Source: CAD feature listing. Evaluate the final solid. Frame: model axes, mm. A direction names the side the tool comes from. Round coordinates to 2 decimals unless told otherwise and drop trailing zeros. Write each loop counter-clockwise with the first axis right and the second up, starting at its lowest first coordinate (ties: lowest second). Pieces come first, ordered by that corner, then holes. Notation, with made-up numbers: (23, 42.5) -> (43, 42.5) arc R22 ccw to (43, 70.5) -> close; hole circle Ø7 at (46.5, -30). An arc over 180 degrees is marked (long way). Put each result on its own line as item: value.
```python
from build123d import *

# Parameters (mm, degrees)
BOSS_EXTRU_1_DEPTH      = 22
D_GAGEMENT_M21_D        = 2.4
ESQUISSE5_W             = 22
ESQUISSE5_H             = 10
BOSS_EXTRU_2_DEPTH      = 5
CONG_1_R                = 10
CONG_3_R                = 1
ENL_V_MAT_EXTRU_2_DEPTH = 3
ESQUISSE12_R            = 1.9376057
ENL_V_MAT_EXTRU_3_DEPTH = 37.235341952
ESQUISSE13_R            = 2.5
ENL_V_MAT_EXTRU_4_DEPTH = 2


with BuildPart() as part:
    # Esquisse1 → Boss.-Extru.1 (new body)
    with BuildSketch(Plane.XY):
        with BuildLine():
            Line((0, 10), (0, 0))
            Line((0, 0), (6, 0))
            ThreePointArc((6, 0), (11, 5), (16, 0))
            Line((16, 0), (22, 0))
            Line((22, 0), (22, 10))
            Line((22, 10), (0, 10))
        make_face()
    extrude(amount=BOSS_EXTRU_1_DEPTH)

    # Dégagement M21 (through all)
    with Locations(Plane(origin=(0, 10, 0), x_dir=(1, 0, 0), z_dir=(0, 1, 0))):
        with Locations((11, -6), (11, -18), (3, -12), (19, -12)):
            Hole(D_GAGEMENT_M21_D / 2)

    # Esquisse5 → Boss.-Extru.2 (add)
    with BuildSketch(Plane.XY.offset(22)):
        with Locations((11, 5)):
            Rectangle(ESQUISSE5_W, ESQUISSE5_H)
    extrude(amount=BOSS_EXTRU_2_DEPTH)

    # Congé1
    # the kernel refuses this fillet: 10 mm, written as the material it takes off along each edge
    with BuildSketch(Plane(origin=(0, 35, 0), x_dir=(0, 0, 1), z_dir=(0, -1, 0))) as cong_1_piece_1:
        with BuildLine():
            CenterArc((CONG_1_R, -CONG_1_R), CONG_1_R, 90, 90)
            Line((0, -CONG_1_R), (0, 0))
            Line((0, 0), (CONG_1_R, 0))
        make_face()
    extrude(amount=60, mode=Mode.SUBTRACT)
    with BuildSketch(Plane(origin=(0, 35, 27), x_dir=(0, 0, -1), z_dir=(0, -1, 0)), Plane(origin=(22, -25, 0), x_dir=(-1, 0, 0), z_dir=(0, 1, 0)), Plane(origin=(22, -25, 27), x_dir=(0, 0, -1), z_dir=(0, 1, 0))) as cong_1_piece_2:
        with BuildLine():
            CenterArc((CONG_1_R, CONG_1_R), CONG_1_R, 180, 90)
            Line((0, CONG_1_R), (0, 0))
            Line((0, 0), (CONG_1_R, 0))
        make_face()
    extrude(amount=60, mode=Mode.SUBTRACT)

    # Congé3
    cong_3_edges = [part.edges().sort_by_distance(p)[0] for p in [
        (11, 10, 0),
        (0, 10, 13.5),
        (11, 10, 27),
        (22, 10, 13.5),
        (19.071067812, 10, 24.071067812),
        (19.071067812, 10, 2.928932188),
        (2.928932188, 10, 24.071067812),
        (2.928932188, 10, 2.928932188),
    ]]
    fillet(cong_3_edges, radius=CONG_3_R)

    # Esquisse10 → Enlèv. mat.-Extru.2 (cut)
    with BuildSketch(Plane(origin=(0, 0, 22), x_dir=(-1, 0, 0), z_dir=(0, 0, -1))):
        with BuildLine():
            Line((-7, 0), (-15, 0))
            ThreePointArc((-15, 0), (-11, 4), (-7, 0))
        make_face()
    extrude(amount=-ENL_V_MAT_EXTRU_2_DEPTH, mode=Mode.SUBTRACT)

    # Esquisse12 → Enlèv. mat.-Extru.3 (cut, through all)
    with BuildSketch(Plane(origin=(0, 10, 0), x_dir=(1, 0, 0), z_dir=(0, 1, 0))):
        with Locations(Location((11, -23, 0), (0, 0, 270))):
            Circle(ESQUISSE12_R)
    extrude(amount=-ENL_V_MAT_EXTRU_3_DEPTH, mode=Mode.SUBTRACT)

    # Esquisse13 → Enlèv. mat.-Extru.4 (cut)
    with BuildSketch(Plane(origin=(0, 10, 0), x_dir=(1, 0, 0), z_dir=(0, 1, 0))):
        with Locations(Location((11, -12, 0), (0, 0, 270))):
            Circle(ESQUISSE13_R)
    extrude(amount=-ENL_V_MAT_EXTRU_4_DEPTH, mode=Mode.SUBTRACT)


solid = part.part
```
Q1. Draft query along X for faces 1 (the cylindrical face through (0.301, 9.715, 13.549)), 2 (the cylindrical face through (19.15, 4.44, 3.01)), 3 (the cylindrical face through (19.95, 4.93, 12.73)). Return one class per face: +X half, -X half, draft (parallel to the pull), parting line (faces both ways), or undercut.
Ans:
face 1: -X half
face 2: +X half
face 3: undercut
Q2. Pin query (flat end, axial travel): pin 1 (3 mm diameter, centred on y = 1.5, z = 20, fed in from -X); pin 2 (3 mm diameter, centred on x = 11, z = 12, fed in from -Y); pin 3 (1 mm diameter, centred on x = 8.5, y = 2.5, fed in from -Z). Return the tip coordinate at first contact, or that it passes through.
Ans:
pin 1: stops at x = 0.11
pin 2: stops at y = 4.77
pin 3: stops at z = 22
Q3. Cut plane A-A on z = 12. Output: boundary loops of the cut face in (x, y).
Ans:
outline: (0, 0) -> (1.8, 0) -> (1.8, 10) -> (1, 10) arc R1 ccw to (0, 9) -> close; (4.2, 0) -> (6, 0) arc R5 cw to (16, 0) -> (17.8, 0) -> (17.8, 10) -> (13.5, 10) -> (13.5, 8) -> (8.5, 8) -> (8.5, 10) -> (4.2, 10) -> close; (20.2, 0) -> (22, 0) -> (22, 9) arc R1 ccw to (21, 10) -> (20.2, 10) -> close
Q4. Cut plane B-B on y = 6. Output: boundary loops of the cut face in (x, z), and give its area (3 significant figures).
Ans:
outline: (0, 10) arc R10 ccw to (10, 0) -> (12, 0) arc R10 ccw to (22, 10) -> (22, 17) arc R10 ccw to (12, 27) -> (10, 27) arc R10 ccw to (0, 17) -> close; hole circle Ø2.4 at (3, 12); hole circle Ø3.88 at (11, 23); hole circle Ø2.4 at (11, 6); hole circle Ø2.4 at (11, 18); hole circle Ø2.4 at (19, 12)
area: 478 mm^2
Q5. Material intervals for line 1 (Z direction, x = 11, y = 7.25); line 2 (X direction, y = 6, z = 12); line 3 (X direction, y = 8.5, z = 11.5), sorted ascending. Write a range as [from, to].
Ans:
line 1: z = [0, 4.8], [7.2, 16.8], [19.2, 21.06], [24.94, 27]
line 2: x = [0, 1.8], [4.2, 17.8], [20.2, 22]
line 3: x = [0, 1.91], [4.09, 8.55], [13.45, 17.91], [20.09, 22]
Q6. Cut plane C-C on x = 11. Output: boundary loops of the cut face in (y, z).
Ans:
outline: (0, 25) -> (4, 25) -> (4, 24.94) -> (10, 24.94) -> (10, 26) arc R1 ccw to (9, 27) -> (0, 27) -> close; (5, 0) -> (9, 0) arc R1 ccw to (10, 1) -> (10, 4.8) -> (5, 4.8) -> close; (5, 7.2) -> (10, 7.2) -> (10, 9.5) -> (8, 9.5) -> (8, 14.5) -> (10, 14.5) -> (10, 16.8) -> (5, 16.8) -> close; (5, 19.2) -> (10, 19.2) -> (10, 21.06) -> (5, 21.06) -> close
Q7. Cut plane D-D on z = 16.5. Output: boundary loops of the cut face in (x, y), and give its area (3 significant figures).
Ans:
outline: (0, 0) -> (6, 0) arc R5 cw to (16, 0) -> (22, 0) -> (22, 9) arc R1 ccw to (21, 10) -> (1, 10) arc R1 ccw to (0, 9) -> close
area: 180 mm^2
Q8. Reachability of faces 4 (the flat face through (11, 8, 12)), 5 (the flat face through (11, 5, 27)), 6 (the flat face through (11, 2, 25)) from +Z, -Z, +X, -X, +Y, -Y: full face, straight path, thin tool, end or side. Return the list, or none.
Ans:
face 4: +Y
face 5: +Z, +X, -X, +Y, -Y
face 6: -Z, -Y
